Input: part model. Units: mm. Frame: model coordinates. A direction names the side the tool comes from. Give positions to 0.01 mm unless a question says otherwise; leave off trailing zeros. Loops run counter-clockwise (first coordinate to the right, second up) from the corner with the lowest first, then second, coordinate; pieces in that order, holes last. Notation, with made-up numbers: (65, -29) - (107, -29) arc R12 cw to (107, -20) - close; hole circle Ø9 at (-29.5, -30). An arc over 180 degrees is marked (long way). One line per question, with ' | ' between items. Start each with the question number.
from build123d import *

# Parameters (mm, degrees)
SKETCH_1_W             = 37.5
SKETCH_1_H             = 2
SM_BASE_FLANGE_1_DEPTH = 150
OTHER_START            = -18.75
OTHER_1_DEPTH          = 37.5
OTHER_1_2_DEPTH        = 37.5


# Read off the part's stored shape, not the designer's step: 绘制的折弯1
# Sheet-metal steps are written as plain solids
with BuildPart() as part:
    # Sketch 1 → 基体-法兰1 (new, symmetric)
    with BuildSketch(Plane(origin=(0, 0, 0), x_dir=(0, 0, -1), z_dir=(1, 0, 0))):
        with Locations((0, -1)):
            Rectangle(SKETCH_1_W, SKETCH_1_H)
    extrude(amount=SM_BASE_FLANGE_1_DEPTH, both=True)

    # Other 1 outline → Other 1 (cut)
    with BuildSketch(Plane.XY.offset(OTHER_START)):
        with BuildLine():
            ThreePointArc((-110.399002398, -2), (-109.417667209, -0.556604688), (-107.7634, 0))
            Line((-107.7634, 0), (-150, 0))
            Line((-150, 0), (-150, -2))
            Line((-150, -2), (-110.399002398, -2))
        make_face()
        with BuildLine():
            Line((150, 0), (107.7634, 0))
            ThreePointArc((107.7634, 0), (109.417667209, -0.556604688), (110.399002398, -2))
            Line((110.399002398, -2), (150, -2))
            Line((150, -2), (150, 0))
        make_face()
    extrude(amount=OTHER_1_DEPTH, mode=Mode.SUBTRACT)

    # Other 1 2 outline → Other 1 2 (add)
    with BuildSketch(Plane.XY.offset(OTHER_START)):
        with BuildLine():
            Line((-107.7634, -2), (-110.399002398, -2))
            ThreePointArc((-110.399002398, -2), (-110.474633029, -2.364854094), (-110.5, -2.7366))
            Line((-110.5, -2.7366), (-110.5, -42.245355099))
            Line((-110.5, -42.245355099), (-108.5, -42.245355099))
            Line((-108.5, -42.245355099), (-108.5, -2.7366))
            ThreePointArc((-108.5, -2.7366), (-108.284254855, -2.215745145), (-107.7634, -2))
        make_face()
        with BuildLine():
            ThreePointArc((110.5, -2.7366), (110.474633029, -2.364854094), (110.399002398, -2))
            Line((110.399002398, -2), (107.7634, -2))
            ThreePointArc((107.7634, -2), (108.284254855, -2.215745145), (108.5, -2.7366))
            Line((108.5, -2.7366), (108.5, -42.245355099))
            Line((108.5, -42.245355099), (110.5, -42.245355099))
            Line((110.5, -42.245355099), (110.5, -2.7366))
        make_face()
    extrude(amount=OTHER_1_2_DEPTH)


solid = part.part
Q1. Section C-C, the plane x = -83. Output: boundary loops of the cut face in (y, z).
Q2. Line query: L1, parallel to X at y = -26, z = -7; L2, parallel to Y at x = 17, z = -7. Output: solid intervals per line, ascending. Write a range as from..to.
Q3. Section B-B, the plane z = -0.5. Output: boundary loops of the cut face in (x, y), plus the area to 3 significant figures.
Q4. Draft query along X for faces 1 (the face through (-110.5, -22, 0)), 2 (the face through (-1, -1, -18.75)), 3 (the face through (2, -2, 0)), 4 (the face through (110.5, -23, 0)). Return one class per face: +X half, -X half, draft (parallel to the pull), parting line (faces both ways), or undercut.
Q5. Access query for faces 5 (the face through (2, 0, 0)), 6 (the face through (-108.5, -23, 0)). Directions: +Z, -Z, +X, -X, +Y, -Y. A direction counts if a zero-diameter tool reaches every point of the face in a straight line with its end or side. Return the directions, or none.
Q6. Section A-A, the plane y = -25. Output: boundary loops of the cut face in (x, z), plus the area to 3 significant figures.
Q7. First-contact query: pin 1 (12 mm diameter, centred on x = 80.5, y = -7, fed in from +Z); pin 2 (3 mm diameter, centred on x = -18, z = -14, fed in from -Y). Flat tips, straight axial feed; report the tip coordinate or a pass-through.
Solved:
1) outline: (-2, -18.75) - (0, -18.75) - (0, 18.75) - (-2, 18.75) - close
2) L1: x = -110.5..-108.5, 108.5..110.5 | L2: y = -2..0
3) outline: (-110.5, -42.25) - (-108.5, -42.25) - (-108.5, -2.74) arc R0.74 cw to (-107.76, -2) - (107.76, -2) arc R0.74 cw to (108.5, -2.74) - (108.5, -42.25) - (110.5, -42.25) - (110.5, -2.74) arc R2.74 ccw to (107.76, 0) - (-107.76, 0) arc R2.74 ccw to (-110.5, -2.74) - close | area: 600 mm²
4) face 1: -X half | face 2: draft | face 3: undercut | face 4: +X half
5) face 5: +Z, -Z, +X, -X, +Y | face 6: +Z, -Z, -Y
6) outline: (-110.5, -18.75) - (-108.5, -18.75) - (-108.5, 18.75) - (-110.5, 18.75) - close; (108.5, -18.75) - (110.5, -18.75) - (110.5, 18.75) - (108.5, 18.75) - close | area: 150 mm²
7) pin 1: stops at z = 18.75 | pin 2: stops at y = -2
